Part model, mm, in its own coordinate system. A direction names the side the tool comes from. Give positions to 0.01 mm unless a question says otherwise; leave off trailing zeros. Write each loop counter-clockwise with the first axis right and the second up, starting at its lowest first coordinate (ties: lowest second). Pieces come first, ordered by that corner, then holes. Notation, with made-up numbers: M 51.25,-29.5 L 105.25,-29.5 A8 cw 105.25,-22.5 Z; hole C 69,61 d3. An arc over 180 degrees is marked long. Answer as CSV lines item,"result". Start each with the question number.
Item 1: 3-axis set-ups, long thin cutter, end or side, ignore diameter. For faces 1 (the cylindrical face through (-0.29, 1.74, 2.23)), 2 (the cylindrical face through (-0.29, -0.99, -2.23)), 3 (the cylindrical face through (2.579, 0.493, 1.978)): which of +Z, -Z, +X, -X, +Y, -Y reach the whole face in a straight line?
Item 2: Band-saw the part on C-C, the plane y = -0.6. List the corners of the cut face in (x, z).
Item 3: Wall check: L1, parallel to Y at x = 2.5, z = -1.5; L2, parallel to Z at x = 2, y = -1.8. Give the ranges that are in metal, low to high. Write a range as from..to.
Item 4: Pin check, flat tip, straight feed: pin 1 (3 mm diameter, centred on y = 1, z = -1.5, fed in from -X). Stop position of the tip, or through.
Item 5: Band-saw the part on D-D, the plane y = 0.15. List the corners of the cut face in (x, z), then the cut area to 3 significant figures.
Item 6: Band-saw the part on B-B, the plane z = 0. List the corners of the cut face in (x, y).
Item 7: Band-saw the part on A-A, the plane x = 0. List the corners of the cut face in (y, z), then the cut area to 4 significant figures.
Autodesk Inventor part; units mm, degrees
ref_plane "YZ Plane" through (0, 0, 0) normal (1, 0, 0) x (0, 1, 0)
ref_plane "XZ Plane" through (0, 0, 0) normal (0, 1, 0) x (-1, 0, 0)
sketch "Sketch1" plane through (0, 0, 0) normal (0, 1, 0) x (-1, 0, 0)
  circle A0 centre (0, 0) radius 3.25
  dimension "d0" = 6.5
extrude "Extrusion1" add sketch "Sketch1" along normal blind 1
sketch "Sketch2" plane through (0, 1, 0) normal (0, 1, 0) x (1, 0, 0)
  circle A0 centre (0, 0) radius 2.25
  dimension "d3" = 4.5
extrude "Extrusion2" add sketch "Sketch2" along normal blind 2
sketch "Sketch3" plane through (0, 0, 0) normal (0, -1, 0) x (1, 0, 0)
  circle A0 centre (0, 0) radius 2.25
extrude "Extrusion3" add sketch "Sketch3" along normal blind 2
sketch "Sketch4" plane through (0, 0, 0) normal (0, 0, 1) x (1, 0, 0)
  point P0 (0, 0)
chamfer "Chamfer1" distance 0.5 angle 45 1 edges at (-2.25, 3, 0)
equation "\"BendRadius\" = Thickness"
equation "\"BendReliefWidth\" = Thickness"
equation "\"BendReliefDepth\" = 0.5 * Thickness"
equation "\"CornerReliefSize\" = 4 * Thickness"
equation "\"MinimumRemnant\" = 2 * Thickness"
equation "\"TransitionRadius\" = BendRadius"
equation "\"JacobiRadiusSize\" = BendRadius"
equation "\"GapSize\" = Thickness"
Output:
1,face 1,"+Y"
1,face 2,"-Y"
1,face 3,"+Y, -Y"
2,outline,"C 0,0 d4.5"
3,L1,"0..1"
3,L2,"-1.03..1.03"
4,pin 1,"x = -3.25"
5,outline,"C 0,0 d6.5"
5,area,"33.2 mm²"
6,outline,"M -3.25,0 L -2.25,0 L -2.25,-2 L 2.25,-2 L 2.25,0 L 3.25,0 L 3.25,1 L 2.25,1 L 2.25,2.5 L 1.75,3 L -1.75,3 L -2.25,2.5 L -2.25,1 L -3.25,1 Z"
7,outline,"M -2,-2.25 L 0,-2.25 L 0,-3.25 L 1,-3.25 L 1,-2.25 L 2.5,-2.25 L 3,-1.75 L 3,1.75 L 2.5,2.25 L 1,2.25 L 1,3.25 L 0,3.25 L 0,2.25 L -2,2.25 Z"
7,area,"24.25 mm²"
